Check sheet for the drawn part. Datum: minimum x, y, z corner. Units: mm. Give positions to 0.01 mm unless a question says otherwise; leave off trailing zeros. Write each loop counter-clockwise with the first axis right and the second up, starting at its lowest first coordinate (ties: lowest second). Pieces come first, ordered by that corner, then holes. Notation, with made-up numbers: M -40,77 L -1,77 A24 ccw -1,111 Z; hole C 6,8 d3. An arc over 180 degrees is marked long. Write item = value, one per line. Start each with the question number.
1) Gauge pin test, flat end, axial feed: pin 1 (12 mm diameter, centred on x = 5.5, z = 9.5, fed in from -Y). Record the tip position at first contact, or that the pin passes through.
2) Sectioned sample at D-D, the plane z = 12.75. Record the cut outline in (x, y), then the cut area to 3 significant figures.
3) Draft check along Y on the marked faces 1, 2, 3 and 4. Enter one of: pulls with the +Y half, pulls with the -Y half, needs draft (parallel to the pull), parting line crosses it, or undercut.
4) Sectioned sample at C-C, the plane x = 6. Record the cut outline in (y, z) (1 decimal), then the cut area to 3 significant figures.
5) Sectioned sample at A-A, the plane x = 13. Record the cut outline in (y, z).
6) Scan lines: L1, parallel to Y at x = 13, z = 21.25; L2, parallel to X at y = 5.5, z = 22; L3, parallel to X at y = 20.75, z = 10 (1 decimal). Record each from-to range of solid material in increasing order.
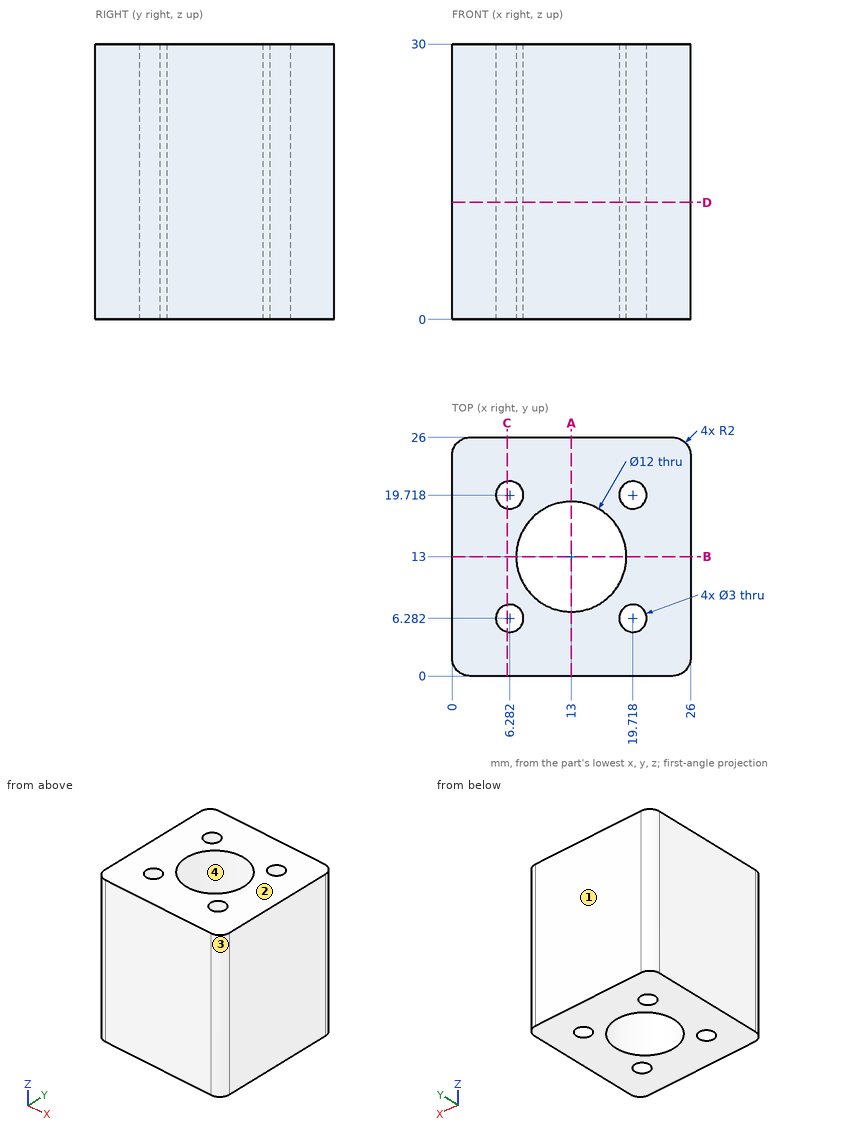
Data:
q1.pin_1 = 0
q2.outline = M 0,2 A2 ccw 2,0 L 24,0 A2 ccw 26,2 L 26,24 A2 ccw 24,26 L 2,26 A2 ccw 0,24 Z; hole C 6.28,6.28 d3; hole C 6.28,19.72 d3; hole C 13,13 d12; hole C 19.72,6.28 d3; hole C 19.72,19.72 d3
q2.area = 531 mm2
q3.face_1 = pulls with the +Y half
q3.face_2 = needs draft
q3.face_3 = pulls with the -Y half
q3.face_4 = undercut
q4.outline = M 0,0 L 4.8,0 L 4.8,30 L 0,30 Z; M 7.8,0 L 18.2,0 L 18.2,30 L 7.8,30 Z; M 21.2,0 L 26,0 L 26,30 L 21.2,30 Z
q4.area = 603 mm2
q5.outline = M 0,0 L 7,0 L 7,30 L 0,30 Z; M 19,0 L 26,0 L 26,30 L 19,30 Z
q6.L1 = 0 to 7, 19 to 26
q6.L2 = 0 to 5, 7.56 to 18.44, 21 to 26
q6.L3 = 0 to 5.2, 7.4 to 18.6, 20.8 to 26
